Source: three-view drawing plus pictorial views. Frame: mm from the lowest corner of the part. A direction names the side the tool comes from. Give positions to 0.01 mm unless a question says otherwise; leave off trailing zeros. Loops run counter-clockwise (first coordinate to the right, second up) from the corner with the lowest first, then second, coordinate; pieces in that order, holes last.
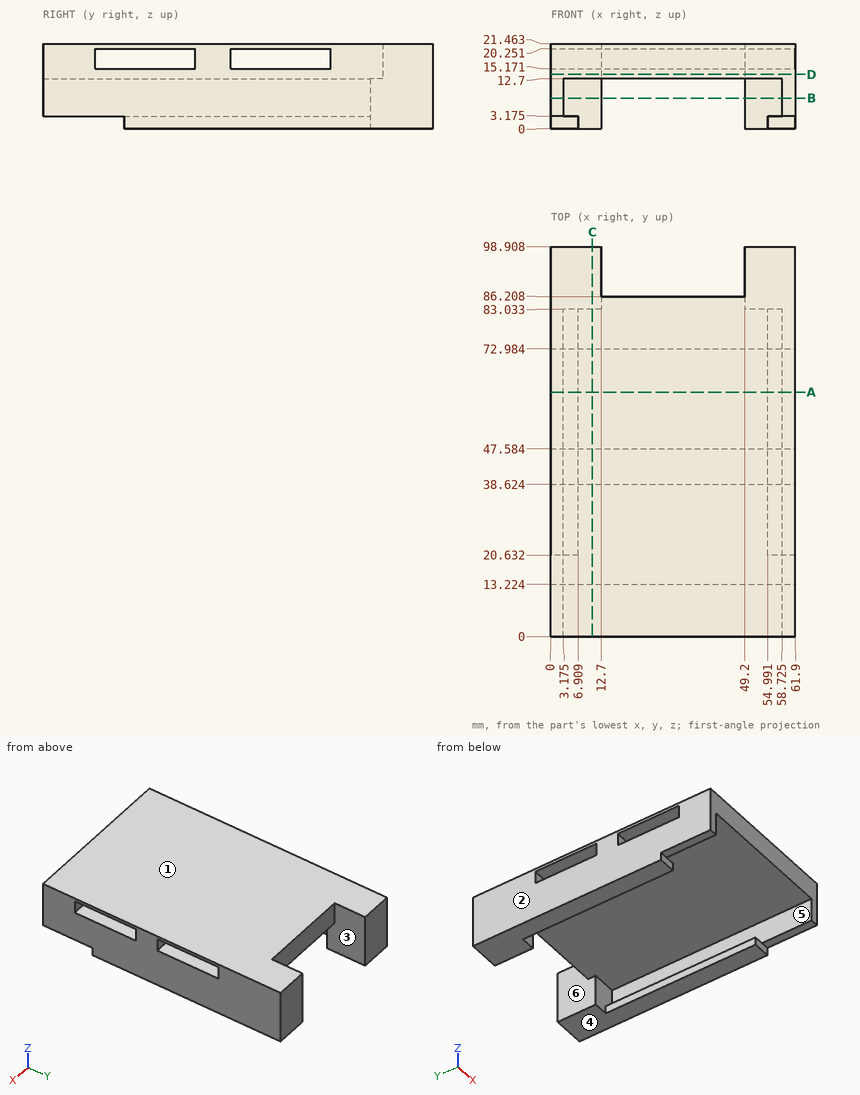
Q1. Section query A-A, the plane y = 62. Return loops of the section in (x, z) (1 decimal).
Q2. Mould query, pull axis X, two halves, no side actions, for the marked faces 1, 2 and 3. Classes: +X half, -X half, draft (parallel to the pull), parting line (faces both ways), or undercut.
Q3. Section query D-D, the plane z = 13.75. Return loops of the section in (x, y), and give its area (3 significant figures).
Q4. Reachability of the marked faces 4, 5 and 6 from +Z, -Z, +X, -X, +Y, -Y: full face, straight path, thin tool, end or side. Return the list, or none.
Q5. Section query B-B, the plane z = 7.75. Return loops of the section in (x, y) (1 decimal).
Q6. Section query C-C, the plane x = 10.5. Return loops of the section in (y, z).
Q7. Pin query (flat end, axial travel): pin 1 Ø3 at (x, y) = (26, 80.5) entering from -Z; pin 2 Ø5 at (x, z) = (7, 8.5) entering from -Y; pin 3 Ø3.5 at (x, z) = (59.5, 1) entering from -Y. Return the tip coordinate at first contact, or that it passes through.
Q8. Material intervals for probe 1 along Y at (x, z) = (15.5, 17); probe 2 along Z at (x, y) = (7.5, 26); probe 3 along X at (y, z) = (21.5, 10) (1 decimal), sorted ascending.
Resolved:
1. outline: (0, 0) - (6.9, 0) - (6.9, 3.2) - (3.2, 3.2) - (3.2, 12.7) - (58.7, 12.7) - (58.7, 3.2) - (55, 3.2) - (55, 0) - (61.9, 0) - (61.9, 15.2) - (0, 15.2) - close; (0, 20.3) - (61.9, 20.3) - (61.9, 21.5) - (0, 21.5) - close
2. face 1: draft
2. face 2: -X half
2. face 3: undercut
3. outline: (0, 0) - (61.9, 0) - (61.9, 98.91) - (49.2, 98.91) - (49.2, 86.21) - (12.7, 86.21) - (12.7, 98.91) - (0, 98.91) - close
3. area: 5,660 mm2
4. face 4: -Z, +X, -X, +Y, -Y
4. face 5: -Y
4. face 6: -Z, +Y
5. outline: (0, 0) - (3.2, 0) - (3.2, 83) - (12.7, 83) - (12.7, 98.9) - (0, 98.9) - close; (49.2, 83) - (58.7, 83) - (58.7, 0) - (61.9, 0) - (61.9, 98.9) - (49.2, 98.9) - close
6. outline: (0, 12.7) - (83.03, 12.7) - (83.03, 0) - (98.91, 0) - (98.91, 21.46) - (0, 21.46) - close; hole (13.22, 15.17) - (38.62, 15.17) - (38.62, 20.25) - (13.22, 20.25) - close; hole (47.58, 15.17) - (72.98, 15.17) - (72.98, 20.25) - (47.58, 20.25) - close
7. pin 1: stops at z = 12.7
7. pin 2: stops at y = 83.03
7. pin 3: stops at y = 20.63
8. probe 1: y = 0 to 13.22, 38.62 to 47.58, 72.98 to 86.21
8. probe 2: z = 12.7 to 15.17, 20.25 to 21.46
8. probe 3: x = 0 to 3.2, 58.7 to 61.9
